Input: part model. Units: mm. Frame: model coordinates. Give positions to 0.01 mm unless a question says otherwise; leave off trailing zeros. Write each loop counter-clockwise with the first axis right and the second up, starting at its lowest first coordinate (ties: lowest second). Pieces come first, ordered by that corner, then holes. Notation, with made-up numbers: (65, -19) -> (90, -19) arc R24 ccw to (90, 12) -> close; hole circle Ø9 at (3, -25). An arc over 180 degrees is marked (long way). Return JSON: item names as keys, results as strings. Group by question number.
Item 1: Section D-D, the plane z = 3.7. Return loops of the section in (x, y), then the cut area to 3 significant figures.
Item 2: Section C-C, the plane y = 15. Return loops of the section in (x, z), then the cut area to 3 significant figures.
Item 3: Pin query (flat end, axial travel): P1, Ø1.5, axis at x = -19.5, z = 3.5, coming from the +Y side; P2, Ø1, axis at x = -24.5, z = 1, coming from the +Y side. Return the tip coordinate at first contact, or that it passes through.
Item 4: Section A-A, the plane x = 0. Return loops of the section in (y, z), then the cut area to 3 significant figures.
Item 5: Mould query, pull axis X, two halves, no side actions, for faces 1 (the face through (-8, 0, 0)), 2 (the face through (-23, -13, 3)), 3 (the face through (-28, 21, 2)). Classes: released by +X, released by -X, zero draft, split by the parting line, or undercut.
Item 6: Line query: line 1 (Y direction, x = 23, z = 1.35); line 2 (X direction, y = -15, z = 1); line 3 (Y direction, x = -22.5, z = 3.2). Output: solid intervals per line, ascending. Write a range as [from, to].
Autodesk Inventor part; units mm, degrees
ref_plane "YZ Plane" through (0, 0, 0) normal (1, 0, 0) x (0, 1, 0)
ref_plane "XZ Plane" through (0, 0, 0) normal (0, 1, 0) x (-1, 0, 0)
ref_plane "XY Plane" through (0, 0, 0) normal (0, 0, 1) x (1, 0, 0)
sketch "Эскиз1" plane through (0, 0, 0) normal (0, 0, 1) x (1, 0, 0)
  circle A0 centre (0, 0) radius 35
  dimension "d7" = 70
extrude "Выдавливание1" add sketch "Эскиз1" along normal blind 5
sketch "Эскиз2" plane through (0, 0, 5) normal (0, 0, 1) x (1, 0, 0)
  circle A0 centre (-23, 15) radius 2
  point P0 (0, 0)
  dimension "d4" = 4
  dimension "d5" = 15
  dimension "d6" = 23
extrude "Выдавливание2" cut sketch "Эскиз2" against normal through all
mirror "Зеркальное отражение1" about plane through (0, 0, 0) normal (0, 1, 0) of "Выдавливание2"
mirror "Зеркальное отражение2" about plane through (0, 0, 0) normal (1, 0, 0) of "Выдавливание2", "Зеркальное отражение1"
sketch "Эскиз19" plane through (0, 0, 5) normal (0, 0, 1) x (1, 0, 0)
  circle A0 centre (0, 0) radius 7.5
  dimension "d75" = 15
extrude "Выдавливание18" cut sketch "Эскиз19" against normal through all
properties part number "000.005.005.001 - ОСНОВАНИЕ" material "Пластик АБС"
Answer below:
{
 "1": {"outline": "circle Ø70 at (0, 0); hole circle Ø4 at (-23, -15); hole circle Ø4 at (-23, 15); hole circle Ø15 at (0, 0); hole circle Ø4 at (23, -15); hole circle Ø4 at (23, 15)", "area": "3,620 mm2"},
 "2": {"outline": "(-31.62, 0) -> (-25, 0) -> (-25, 5) -> (-31.62, 5) -> close; (-21, 0) -> (21, 0) -> (21, 5) -> (-21, 5) -> close; (25, 0) -> (31.62, 0) -> (31.62, 5) -> (25, 5) -> close", "area": "276 mm2"},
 "3": {"P1": "stops at y = 29.55", "P2": "stops at y = 25.48"},
 "4": {"outline": "(-35, 0) -> (-7.5, 0) -> (-7.5, 5) -> (-35, 5) -> close; (7.5, 0) -> (35, 0) -> (35, 5) -> (7.5, 5) -> close", "area": "275 mm2"},
 "5": {"face 1": "zero draft", "face 2": "undercut", "face 3": "split by the parting line"},
 "6": {"line 1": "y = [-26.38, -17], [-13, 13], [17, 26.38]", "line 2": "x = [-31.62, -25], [-21, 21], [25, 31.62]", "line 3": "y = [-26.81, -16.94], [-13.06, 13.06], [16.94, 26.81]"}
}
